CAD build for the part. Positions are in the model's coordinates, mm. Face numbers are marked on the shaded views. A direction names the side the tool comes from. Round coordinates to 2 decimals unless told otherwise and drop trailing zeros. Order: outer loops, then holes, each group sorted by start corner. A loop starts at its lowest first (then second) coordinate and runs counter-clockwise, first axis right, second up. Notation, with made-up numbers: (34, 64.5) -> (58, 64.5) arc R38 cw to (58, 103.5) -> close; hole circle Ø3 at (-14.5, -21). An arc over 180 degrees is marked (long way). Return JSON: item names as keys, results as strings. Group by question number.
Q1. Cut at A-A (x = 7.5). Write the cut outline in (y, z).
Q2. Which spindle directions (+Z, -Z, +X, -X, +Y, -Y) get a long thin tool onto all of the face, cutting with end or side? Do the marked faces 4, 5 and 6. Say none if no direction does.
Q3. Probe line 1 along X through (y, z) = (-0.5, 3); line 2 along Y through (x, z) = (3, 4.5). List the from-to ranges inside material, lowest first.
Q4. Flat gauge pins, fed straight in: pin 1 (6 mm diameter, centred on x = 10.5, z = -0.5, fed in from -Y); pin 2 (1 mm diameter, centred on y = -2, z = -4, fed in from +X); pin 3 (1 mm diameter, centred on y = 1.5, z = 1, fed in from -X). Where does each tip first touch, or does it go through?
Q5. Mould opens along Z. For the marked faces 1, 2 and 3 say: +Z half, -Z half, draft (parallel to the pull), parting line (faces both ways), or undercut.
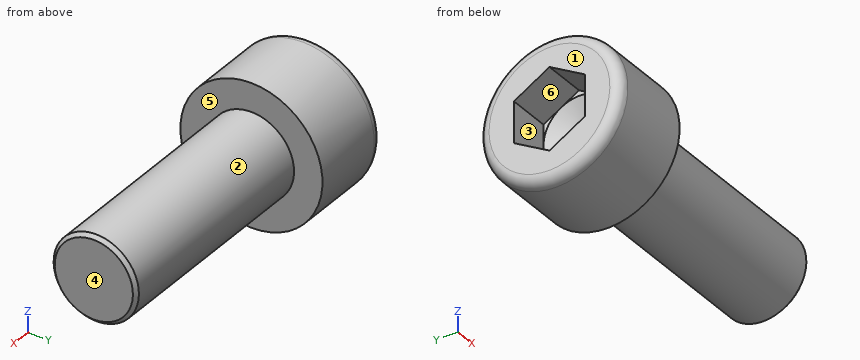
from build123d import *

# Parameters (mm, degrees)
SKETCH1_R           = 5
BASEHEAD_DEPTH      = 6
SKETCH2_R           = 3
BASEBODY_DEPTH      = 16
HEXAGONSOCKET_DEPTH = 3
TOPFILLET_R         = 0.75
CHAMFER1_SIZE       = 0.25


with BuildPart() as part:
    # Sketch1 → BaseHead (new body)
    with BuildSketch(Plane(origin=(0, 0, 0), x_dir=(0, 0, -1), z_dir=(1, 0, 0))):
        Circle(SKETCH1_R)
    extrude(amount=BASEHEAD_DEPTH)

    # Sketch2 → BaseBody (add)
    with BuildSketch(Plane(origin=(6, 0, 0), x_dir=(0, 0, -1), z_dir=(1, 0, 0))):
        Circle(SKETCH2_R)
    extrude(amount=BASEBODY_DEPTH)

    # Sketch3 → HexagonSocket (cut)
    with BuildSketch(Plane(origin=(0, 0, 0), x_dir=(0, 0, -1), z_dir=(1, 0, 0))):
        Polygon((2.886751346, 0), (1.443375673, 2.5), (-1.443375673, 2.5), (-2.886751346, 0), (-1.443375673, -2.5), (1.443375673, -2.5), align=None)
    extrude(amount=HEXAGONSOCKET_DEPTH, mode=Mode.SUBTRACT)

    # Sketch4 → Cut-Revolve1 (revolve, cut)
    with BuildSketch(Plane(origin=(-4.19613823, 0.75, 0), x_dir=(-1, 0, 0), z_dir=(0, 0, 1))):
        Polygon((-7.19613823, 3.25), (-8.639513903, 0.75), (-7.19613823, 0.75), align=None)
    revolve(axis=Axis((0.838992387, 0, 0), (-1, 0, 0)), mode=Mode.SUBTRACT)

    # TopFillet
    topfillet_edges = [part.edges().sort_by_distance(p)[0] for p in [
        (0, 0, 5),
    ]]
    fillet(topfillet_edges, radius=TOPFILLET_R)

    # Chamfer1
    chamfer1_edges = [part.edges().sort_by_distance(p)[0] for p in [
        (22, 0, 3),
    ]]
    chamfer(chamfer1_edges, length=CHAMFER1_SIZE)


solid = part.part
Solution:
{
 "1": {"outline": "circle Ø6 at (0, 0)"},
 "2": {"face 4": "+Z, -Z, +X, +Y, -Y", "face 5": "+X", "face 6": "-X"},
 "3": {"line 1": "x = 0 to 6", "line 2": "y = -2.18 to 2.18"},
 "4": {"pin 1": "stops at y = -3", "pin 2": "stops at x = 6", "pin 3": "stops at x = 3.11"},
 "5": {"face 1": "draft", "face 2": "parting line", "face 3": "undercut"}
}
